The listing builds one solid part. Answer for the finished solid, in the listing's coordinates (mm). Face numbers are marked on the shaded views. Coordinates: 2 decimals unless noted, no trailing zeros. Write each loop counter-clockwise with the first axis right and the second up, starting at its lowest first coordinate (ties: lowest second). Pieces come first, ordered by that corner, then holes.
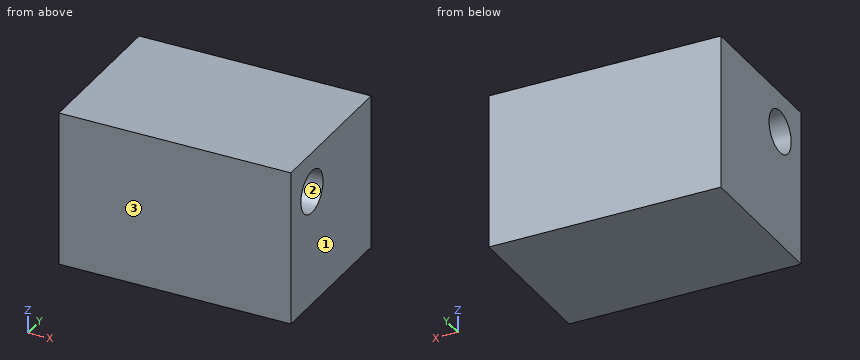
from build123d import *

# Parameters (mm, degrees)
F0_W     = 38.1
F0_H     = 25.4
F1_DEPTH = 25.4
F3_D     = 7


with BuildPart() as f1:
    # F0 (on Top) → F1 (new body)
    with BuildSketch(Plane.XY):
        with Locations((19.05, 12.7)):
            Rectangle(F0_W, F0_H)
    extrude(amount=F1_DEPTH)

    # F3 (through all)
    with Locations(Plane.YZ.offset(38.1)):
        with Locations((6.66, 18.852)):
            Hole(F3_D / 2)


solid = f1.part
1. Section C-C on x = 9 is taken. Give the vertices of the cut face in (y, z), then the cut area to 3 significant figures.
Results found:
outline: (0, 0) - (25.4, 0) - (25.4, 25.4) - (0, 25.4) - close; hole circle Ø7 at (6.66, 18.85)
area: 607 mm2
2. For a pull along Y with two mould halves and no side action, classify the marked faces 1, 2 and 3 as pulls with the +Y half, pulls with the -Y half, needs draft (parallel to the pull), parting line crosses it, or undercut.
Results found:
face 1: needs draft
face 2: undercut
face 3: pulls with the -Y half
3. Section A-A on y = 6.66 is taken. Give the vertices of the cut face in (x, z).
Results found:
outline: (0, 0) - (38.1, 0) - (38.1, 15.35) - (0, 15.35) - close; (0, 22.35) - (38.1, 22.35) - (38.1, 25.4) - (0, 25.4) - close
4. Section B-B on z = 19.75 is taken. Give the vertices of the cut face in (x, y).
Results found:
outline: (0, 0) - (38.1, 0) - (38.1, 3.28) - (0, 3.28) - close; (0, 10.04) - (38.1, 10.04) - (38.1, 25.4) - (0, 25.4) - close
5. Find the intervals of material crossed by L1, parallel to Z at x = 27.5, y = 6.66; L2, parallel to Z at x = 27, y = 4; L3, parallel to Y at x = 27.5, z = 20.25, in increasing order.
Results found:
L1: z = 0 to 15.35, 22.35 to 25.4
L2: z = 0 to 16.58, 21.13 to 25.4
L3: y = 0 to 3.45, 9.87 to 25.4
